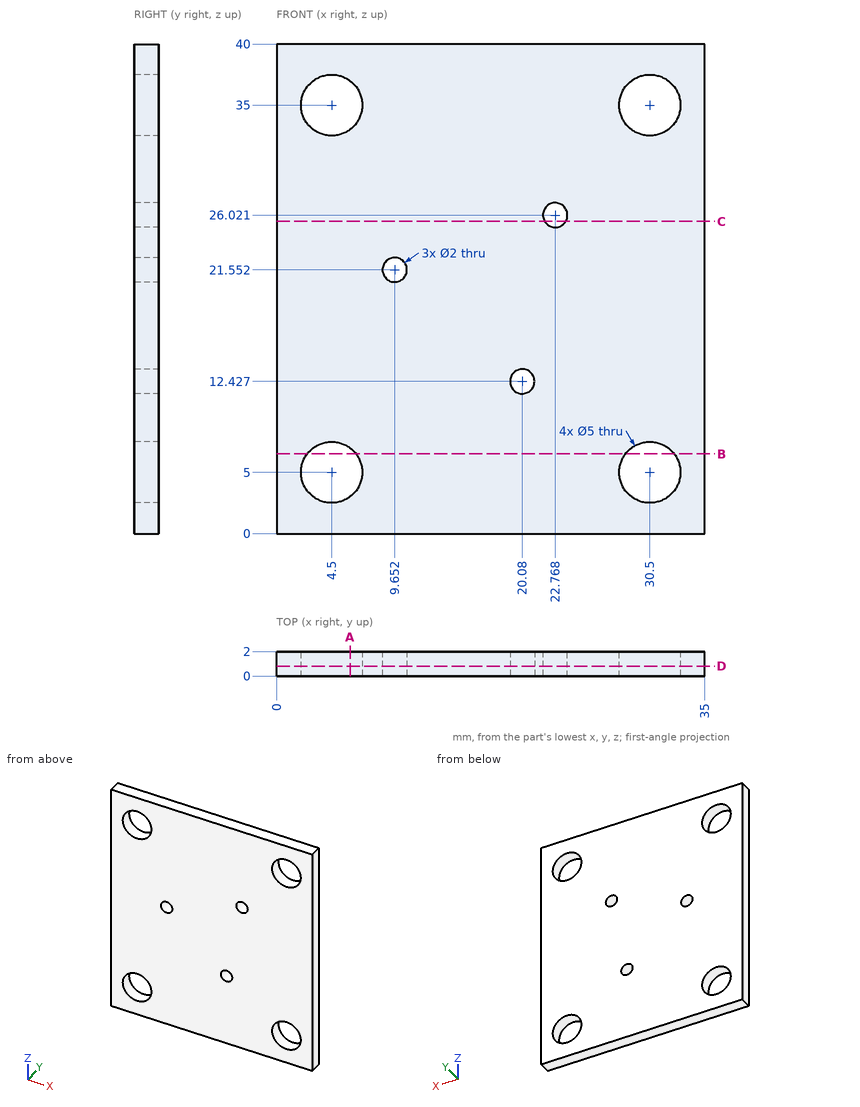
Geometry: see drawing. Coordinates: mm, zero at the bounding-box minimum. Give positions to 0.01 mm unless a question says otherwise; leave off trailing zeros. Order: outer loops, then holes, each group sorted by start corner. A loop starts at its lowest first (then second) coordinate and runs counter-clockwise, first axis right, second up.
Q1. Section C-C on z = 25.5. Output: boundary loops of the cut face in (x, y) (1 decimal).
Checked values:
outline: (0, 0) - (21.9, 0) - (21.9, 2) - (0, 2) - close; (23.6, 0) - (35, 0) - (35, 2) - (23.6, 2) - close
Q2. Ray query, probe 1 along Z at (x, y) = (30.5, 1.1); probe 2 along Z at (x, y) = (5, 1.7); probe 3 along X at (y, z) = (0.65, 3.5). Return the intervals inside material, ascending.
Checked values:
probe 1: z = 0 to 2.5, 7.5 to 32.5, 37.5 to 40
probe 2: z = 0 to 2.55, 7.45 to 32.55, 37.45 to 40
probe 3: x = 0 to 2.5, 6.5 to 28.5, 32.5 to 35
Q3. Section D-D on y = 0.8. Output: boundary loops of the cut face in (x, z).
Checked values:
outline: (0, 0) - (35, 0) - (35, 40) - (0, 40) - close; hole circle Ø5 at (4.5, 5); hole circle Ø5 at (4.5, 35); hole circle Ø2 at (9.65, 21.55); hole circle Ø2 at (20.08, 12.43); hole circle Ø2 at (22.77, 26.02); hole circle Ø5 at (30.5, 5); hole circle Ø5 at (30.5, 35)
Q4. Section A-A on x = 6. Output: boundary loops of the cut face in (y, z).
Checked values:
outline: (0, 0) - (2, 0) - (2, 3) - (0, 3) - close; (0, 7) - (2, 7) - (2, 33) - (0, 33) - close; (0, 37) - (2, 37) - (2, 40) - (0, 40) - close
Q5. Section B-B on z = 6.5. Output: boundary loops of the cut face in (x, y).
Checked values:
outline: (0, 0) - (2.5, 0) - (2.5, 2) - (0, 2) - close; (6.5, 0) - (28.5, 0) - (28.5, 2) - (6.5, 2) - close; (32.5, 0) - (35, 0) - (35, 2) - (32.5, 2) - close
